from build123d import *

# Parameters (mm, degrees)
F0_W     = 101.6
F0_H     = 98.425
F1_DEPTH = 3.175
F3_D     = 5.1054
F3_DEPTH = 25
F3_TIP   = 1.5338169022


# Not quite as in the source:
# - a length typed as a fraction of an inch, garbled in the dataset ("3 / 203.2 mm" for 3/8 in), is restored


with BuildPart() as f1:
    # F0 (on Right) → F1 (new body)
    with BuildSketch(Plane.YZ):
        Rectangle(F0_W, F0_H)
    extrude(amount=F1_DEPTH)

    # F3
    with Locations(Plane.YZ.offset(3.175)):
        with Locations((0, -19.05), (20.6375, 0)):
            Hole(F3_D / 2, depth=F3_DEPTH)
            with Locations((0, 0, -(F3_DEPTH + F3_TIP / 2))):  # 118° drill point
                Cone(0, F3_D / 2, F3_TIP, mode=Mode.SUBTRACT)


solid = f1.part
Source: CAD feature listing. Evaluate the final solid. Frame: model axes, mm. Coordinates: 2 decimals unless noted, no trailing zeros. Loops run counter-clockwise (first coordinate to the right, second up) from the corner with the lowest first, then second, coordinate; pieces in that order, holes last. Notation, with made-up numbers: (-5, -10) - (51, -10) arc R27 cw to (51, 6) - close; hole circle Ø3 at (-23, 33). An arc over 180 degrees is marked (long way). One line per question, with ' | ' between items.
1) Section B-B, the plane z = 0. Return loops of the section in (x, y) (3 decimals).
Report:
outline: (0, -50.8) - (3.175, -50.8) - (3.175, 18.085) - (0, 18.085) - close; (0, 23.19) - (3.175, 23.19) - (3.175, 50.8) - (0, 50.8) - close
2) Section A-A, the plane y = 0. Return loops of the section in (x, z) (1 decimal), then the cut area to 3 significant figures.
Report:
outline: (0, -49.2) - (3.2, -49.2) - (3.2, -21.6) - (0, -21.6) - close; (0, -16.5) - (3.2, -16.5) - (3.2, 49.2) - (0, 49.2) - close | area: 296 mm²
3) Pull-direction query (Z, two-part tool) for faces 1 (the face through (2, 50.8, -1)), 2 (the face through (1.565, -1.372, -16.898)), 3 (the face through (2, -1, -49.212)); classes: released by +Z, released by -Z, zero draft, split by the parting line, or undercut.
Report:
face 1: zero draft | face 2: undercut | face 3: released by -Z
4) First-contact query: P1, Ø4, axis at y = -33.5, z = -13, coming from the -X side. Flat tip, straight axial feed; report the tip coordinate or a pass-through.
Report:
P1: stops at x = 0
5) Line query: line 1 along Z through (x, y) = (2.55, 0); line 2 along Z through (x, y) = (0.75, 1.5). Output: solid intervals per line, ascending.
Report:
line 1: z = -49.21 to -21.6, -16.5 to 49.21 | line 2: z = -49.21 to -21.12, -16.98 to 49.21
